```python
from build123d import *

# Parameters (mm, degrees)
SKETCH_W        = 137
SKETCH_H        = 42.62
SKETCH_R        = 2.5
SKETCH_W_2      = 3
SKETCH_H_2      = 7
PAD_DEPTH       = 24.7
SKETCH001_W     = 125
SKETCH001_H     = 30.62
POCKET_DEPTH    = 18.7
POCKET001_DEPTH = 2
POCKET002_DEPTH = 24.7
SKETCH004_W     = 1.7
SKETCH004_H     = 2
SKETCH004_W_2   = 2
SKETCH004_H_2   = 1.7
POCKET003_DEPTH = 127


with BuildPart() as part:
    # Sketch → Pad (new body)
    with BuildSketch(Plane.XY):
        Rectangle(SKETCH_W, SKETCH_H)
        with Locations((30, 9.81)):
            Circle(SKETCH_R, mode=Mode.SUBTRACT)
        with Locations((-30, 9.81)):
            Circle(SKETCH_R, mode=Mode.SUBTRACT)
        with Locations((-56, -5.81)):
            Rectangle(SKETCH_W_2, SKETCH_H_2, mode=Mode.SUBTRACT)
    extrude(amount=PAD_DEPTH)

    # Sketch001 (on Face12 of Pad) → Pocket (cut)
    with BuildSketch(Plane.XY.offset(24.7)):
        Rectangle(SKETCH001_W, SKETCH001_H)
    extrude(amount=-POCKET_DEPTH, mode=Mode.SUBTRACT)

    # Sketch002 (on Face17 of Pocket) → Pocket001 (cut)
    with BuildSketch(Plane.XY.offset(6)):
        Polygon((-26, 7.500599), (-26, 12.119401), (-30, 14.428802), (-34, 12.119401), (-34, 7.500599), (-30, 5.191198), align=None)
        Polygon((34, 7.500599), (34, 12.119401), (30, 14.428802), (26, 12.119401), (26, 7.500599), (30, 5.191198), align=None)
    extrude(amount=-POCKET001_DEPTH, mode=Mode.SUBTRACT)

    # Sketch003 (on Face5 of Pocket001) → Pocket002 (cut)
    with BuildSketch(Plane.XY.offset(24.7)):
        Polygon((62.5, 21.31), (68.5, 21.31), (68.5, -21.31), (62.5, -21.31), (62.5, -19.16), (64.5, -19.16), (64.5, -17.46), (62.5, -17.46), (62.5, -15.31), (62.5, 15.31), (62.5, 17.46), (64.5, 17.46), (64.5, 19.16), (62.5, 19.16), align=None)
    extrude(amount=-POCKET002_DEPTH, mode=Mode.SUBTRACT)

    # Sketch004 (on Face9 of Pocket002) → Pocket003 (cut)
    with BuildSketch(Plane.YZ.offset(64.5)):
        with Locations((-18.31, 23.7)):
            Rectangle(SKETCH004_W, SKETCH004_H)
        with Locations((18.31, 23.7)):
            Rectangle(SKETCH004_W, SKETCH004_H)
        with Locations((-16.31, 13.85)):
            Rectangle(SKETCH004_W_2, SKETCH004_H_2)
        with Locations((16.31, 13.85)):
            Rectangle(SKETCH004_W_2, SKETCH004_H_2)
    extrude(amount=-POCKET003_DEPTH, mode=Mode.SUBTRACT)


solid = part.part
```
The listing builds one solid part. Answer for the finished solid, in the listing's coordinates (mm). A direction names the side the tool comes from. Give positions to 0.01 mm unless a question says otherwise; leave off trailing zeros. Order: outer loops, then holes, each group sorted by start corner. A loop starts at its lowest first (then second) coordinate and runs counter-clockwise, first axis right, second up. Notation, with made-up numbers: (-13, 53) - (31, 53) arc R17 cw to (31, 83) - close; hole circle Ø8 at (36, 55.5). An arc over 180 degrees is marked (long way). Use one line per item in the form item = value. Start each with the question number.
(1) A cutting plane is placed at C-C, the plane z = 7.75. Write down the section's boundary in (x, y), then the cut area to 3 significant figures.
(2) The mould has two halves that part along Y. Classify faces 6 (the flat face through (32, 8, 4)), 7 (the flat face through (-1, -15.31, 10)), 8 (the flat face through (-4, 21.31, 12)), 9 (the flat face through (-3, 0, 0)): released by +Y, released by -Y, zero draft, split by the parting line, or undercut.
(3) Consider line 1 (X direction, y = 9.81, z = 1.7); line 2 (Y direction, x = -17, z = 21); line 3 (Y direction, x = 30, z = 1.8). Determine where each line is inside the solid, lowest interval first. Write a range as from..to.
(4) A cutting plane is placed at B-B, the plane x = 14.5. Write down the section's boundary in (y, z), then the cut area to 3 significant figures.
(5) A cutting plane is placed at D-D, the plane y = 3. Write down the section's boundary in (x, z).
(6) A cutting plane is placed at A-A, the plane y = 9.81. Write down the section's boundary in (x, z).
(7) Flat-ended cylindrical pins translate along their axes: pin 1 Ø2 at (y, z) = (0, 5) entering from +X; pin 2 Ø2 at (x, z) = (63, 13) entering from +Y; pin 3 Ø24.5 at (x, y) = (-21, 2) entering from +Z; pin 4 Ø1 at (y, z) = (3, 7) entering from +X. Find the tip coordinate at first contact, or state that the pin passes through.
(8) For faces 1 (the flat face through (62.5, -1, 5)), 2 (the flat face through (-1, 15.31, 10)), 3 (the flat face through (62.5, 20, 13)), 4 (the flat face through (-28, 8, 4)), 5 (the cylindrical face through (28.16, 11.5, 1.97)), determine the directions among +Z, -Z, +X, -X, +Y, -Y from which every point of the face is accessible in a straight line to the end or side of a thin tool.
Ans:
q1.outline = (-68.5, -21.31) - (62.5, -21.31) - (62.5, -19.16) - (64.5, -19.16) - (64.5, -17.46) - (62.5, -17.46) - (62.5, -15.31) - (-62.5, -15.31) - (-62.5, 15.31) - (62.5, 15.31) - (62.5, 17.46) - (64.5, 17.46) - (64.5, 19.16) - (62.5, 19.16) - (62.5, 21.31) - (-68.5, 21.31) - close
q1.area = 1,760 mm^2
q2.face_6 = undercut
q2.face_7 = undercut
q2.face_8 = released by +Y
q2.face_9 = zero draft
q3.line_1 = -68.5..-32.5, -27.5..27.5, 32.5..62.5
q3.line_2 = -21.31..-15.31, 15.31..21.31
q3.line_3 = -21.31..7.31, 12.31..21.31
q4.outline = (-21.31, 0) - (21.31, 0) - (21.31, 24.7) - (19.16, 24.7) - (19.16, 22.7) - (17.46, 22.7) - (17.46, 24.7) - (15.31, 24.7) - (15.31, 14.7) - (17.31, 14.7) - (17.31, 13) - (15.31, 13) - (15.31, 6) - (-15.31, 6) - (-15.31, 13) - (-17.31, 13) - (-17.31, 14.7) - (-15.31, 14.7) - (-15.31, 24.7) - (-17.46, 24.7) - (-17.46, 22.7) - (-19.16, 22.7) - (-19.16, 24.7) - (-21.31, 24.7) - close
q4.area = 467 mm^2
q5.outline = (-68.5, 0) - (62.5, 0) - (62.5, 6) - (-62.5, 6) - (-62.5, 24.7) - (-68.5, 24.7) - close
q6.outline = (-68.5, 0) - (-32.5, 0) - (-32.5, 4) - (-34, 4) - (-34, 6) - (-62.5, 6) - (-62.5, 24.7) - (-68.5, 24.7) - close; (-27.5, 0) - (27.5, 0) - (27.5, 4) - (26, 4) - (26, 6) - (-26, 6) - (-26, 4) - (-27.5, 4) - close; (32.5, 0) - (62.5, 0) - (62.5, 6) - (34, 6) - (34, 4) - (32.5, 4) - close
q7.pin_1 = 62.5
q7.pin_2 = 21.31
q7.pin_3 = 6
q7.pin_4 = -62.5
q8.face_1 = +Z, -Z, +X
q8.face_2 = +Z, +X
q8.face_3 = +Z, -Z, +X, +Y
q8.face_4 = +Z
q8.face_5 = +Z, -Z
